Part model, mm, in its own coordinate system. A direction names the side the tool comes from. Round coordinates to 2 decimals unless told otherwise and drop trailing zeros. Loops run counter-clockwise (first coordinate to the right, second up) from the corner with the lowest first, then second, coordinate; pieces in that order, holes last. Notation, with made-up numbers: (-34, 37) - (17, 37) arc R14 ccw to (17, 50) - close; hole circle Ø6 at (-26.5, 4.5). An arc over 180 degrees is marked (long way). Write each question's results on one line, items separated by ' | '. Start each with the question number.
(1) Flat gauge pins, fed straight in: P1, Ø1, axis at x = 7, y = -0.5, coming from the +Z side; P2, Ø1.1, axis at x = -6.5, y = 6.5, coming from the +Z side; P3, Ø5, axis at x = 25, z = 7, coming from the -Y side. Where does each tip first touch, or does it go through?
(2) Cut at A-A, the plane z = 7. List the corners of the cut face in (x, y), then the cut area to 3 significant figures.
(3) Drill centre lines: L1, parallel to Y at x = -23.5, z = 11; L2, parallel to Z at x = 25, y = 6.8; L3, parallel to Y at x = -18, z = 0.45. Where is each one in solid material? Low to high.
(4) Cut at B-B, the plane x = 18. List the corners of the cut face in (y, z), then the cut area to 3 significant figures.
(5) Mould opens along Y. For faces 4 (the face through (-19.75, -0.08, 0.49)), 5 (the face through (-0.42, 5.715, 1.301)), 6 (the face through (23.8, 7, 9.3)), 7 (the face through (0.3, 6.5, 2)) say: released by +Y, released by -Y, zero draft, split by the parting line, or undercut.
(6) Cut at D-D, the plane x = 25. List the corners of the cut face in (y, z).
(7) Tool access for faces 1 (the face through (30, 6.4, 3.3)), 2 (the face through (20, 6.5, 7.1)), 3 (the face through (22.7, 6, 5.8)): list every direction of +Z, -Z, +X, -X, +Y, -Y with a clear straight run to the whole face (end or side of a thin tool).
(8) Cut at C-C, the plane y = -0.75. List the corners of the cut face in (x, z), then the cut area to 3 significant figures.
Autodesk Inventor part; units mm, degrees
ref_plane "YZ Plane" through (0, 0, 0) normal (1, 0, 0) x (0, 1, 0)
ref_plane "XZ Plane" through (0, 0, 0) normal (0, 1, 0) x (-1, 0, 0)
ref_plane "XY Plane" through (0, 0, 0) normal (0, 0, 1) x (1, 0, 0)
sketch "Sketch1" plane through (0, 0, 0) normal (0, 0, 1) x (1, 0, 0)
  line L0 (-30, 5) -> (30, 5)
  line L1 (30, 5) -> (30, -5)
  line L2 (30, -5) -> (-30, -5)
  line L3 (-30, -5) -> (-30, 5)
  line L4 (-30, 5) -> (30, -5) construction
  line L5 (30, 5) -> (-30, -5) construction
  circle A0 centre (-18, 0) radius 1.75
  line L6 (0, 0) -> (0, -5.5046) construction
  circle A1 centre (18, 0) radius 1.75
  dimension "d0" = 60
  dimension "d1" = 10
  dimension "d2" = 3.5
  dimension "d3" = 36
  dimension "d4" = 5
extrude "Plate1" add sketch "Sketch1" along normal blind 1
sketch "Sketch2" plane through (-30, 6, 2) normal (0, 1, 0) x (-1, 0, 0)
  line L0 (-60, 0) -> (0, 0)
  line L1 (0, 0) -> (0, 10)
  line L2 (0, 10) -> (-60, 10)
  line L3 (-60, 10) -> (-60, 0)
edge flange "Flange1" height 12 angle 90 thickness 1 bend radius 1 thickness toward (0, 1, 0) relief tear relief width 1 relief depth 0.5 edges at (0, 5, 1) wall of the first edge with corners at (30, 6, 2) (-30, 6, 2) (-30, 6, 12) (30, 6, 12)
bend "Bend1"
corner "Corner1"
sketch "Sketch3" plane through (-30, 6, 12) normal (0, -1, 0) x (1, 0, 0)
  circle A0 centre (55, -5) radius 2.25
  circle A1 centre (5, -5) radius 2.25
  line L0 (30, -12) -> (30, 5.1941) construction
  line L1 (60, -11) -> (0, -11) construction
  dimension "d20" = 4.5
  dimension "d21" = 4.5
  dimension "d22" = 50
  dimension "d23" = 6
extrude "Cut1" cut sketch "Sketch3" against normal blind 1
sketch "Sketch4" plane through (-30, 7, 12) normal (0, 1, 0) x (1, 0, 0)
  line L0 (60, 0) -> (0, 0)
  line L1 (50, 10) -> (10, 10)
  line L2 (10, 10) -> (10, 0)
  line L3 (10, 0) -> (50, 0)
  line L4 (50, 0) -> (50, 10)
  line L5 (50, 10) -> (10, 0) construction
  line L6 (10, 10) -> (50, 0) construction
  line L7 (60, 10) -> (0, 10)
  point P0 (30, 12)
  point P1 (30, 5)
  dimension "d26" = 40
extrude "Cut2" cut sketch "Sketch4" against normal blind 1
equation "\"d20\" = d21"
equation "\"d24\" = 厚度"
equation "\"d27\" = 厚度"
equation "\"d9\" = 厚度"
equation "\"d10\" = 折彎離隙寬度"
equation "\"d11\" = 折彎離隙深度"
equation "\"d12\" = 最小剩餘"
equation "\"d13\" = 轉移半徑"
equation "\"d16\" = 折彎半徑"
equation "\"d17\" = 轉角離隙大小"
equation "\"d18\" = 間隙大小"
equation "\"d19\" = Jacobi半徑大小"
equation "\"折彎半徑\" = 厚度"
equation "\"折彎離隙寬度\" = 厚度"
equation "\"折彎離隙深度\" = 0.5 * 厚度"
equation "\"轉角離隙大小\" = 4 * 厚度"
equation "\"最小剩餘\" = 2 * 厚度"
equation "\"轉移半徑\" = 折彎半徑"
equation "\"Jacobi半徑大小\" = 折彎半徑"
equation "\"間隙大小\" = 厚度"
properties part number "fan_fix_plate_connect"
A:
1) P1: z = 1 | P2: z = 2 | P3: y = 6
2) outline: (-30, 6) - (-27.25, 6) - (-27.25, 7) - (-30, 7) - close; (-22.75, 6) - (-20, 6) - (-20, 7) - (-22.75, 7) - close; (20, 6) - (22.75, 6) - (22.75, 7) - (20, 7) - close; (27.25, 6) - (30, 6) - (30, 7) - (27.25, 7) - close | area: 11.0 mm2
3) L1: 6 to 7 | L2: 1.13 to 4.75, 9.25 to 12 | L3: -5 to -1.75, 1.75 to 6.26
4) outline: (-5, 0) - (-1.75, 0) - (-1.75, 1) - (-5, 1) - close; (1.75, 0) - (5, 0) arc R2 ccw to (7, 2) - (6, 2) arc R1 cw to (5, 1) - (1.75, 1) - close | area: 8.86 mm2
5) face 4: undercut | face 5: released by -Y | face 6: released by +Y | face 7: zero draft
6) outline: (-5, 0) - (5, 0) arc R2 ccw to (7, 2) - (7, 4.75) - (6, 4.75) - (6, 2) arc R1 cw to (5, 1) - (-5, 1) - close; (6, 9.25) - (7, 9.25) - (7, 12) - (6, 12) - close
7) face 1: +Z, -Z, +X, +Y, -Y | face 2: +Z, +Y, -Y | face 3: +Z, +X, -X, -Y
8) outline: (-30, 0) - (-19.58, 0) - (-19.58, 1) - (-30, 1) - close; (-16.42, 0) - (16.42, 0) - (16.42, 1) - (-16.42, 1) - close; (19.58, 0) - (30, 0) - (30, 1) - (19.58, 1) - close | area: 53.7 mm2
